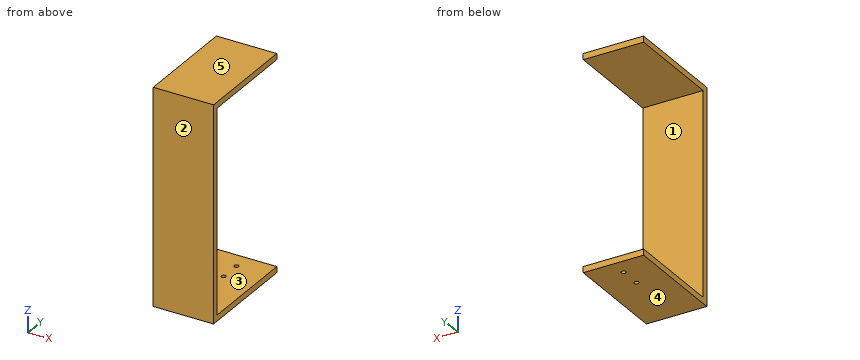
Autodesk Inventor part; units mm, degrees
ref_plane "YZ Plane" through (0, 0, 0) normal (1, 0, 0) x (0, 1, 0)
ref_plane "XZ Plane" through (0, 0, 0) normal (0, 1, 0) x (-1, 0, 0)
ref_plane "XY Plane" through (0, 0, 0) normal (0, 0, 1) x (1, 0, 0)
sketch "Sketch1" plane through (0, 0, 0) normal (0, 1, 0) x (-1, 0, 0)
  line L0 (0, 0) -> (-20, 0)
  line L1 (-20, 0) -> (-20, -67.262)
  line L2 (-20, -67.262) -> (0, -67.262)
  line L3 (0, -67.262) -> (0, 0)
  dimension "d0" = 20
  dimension "d1" = 67.262
extrude "Extrusion1" add sketch "Sketch1" along normal blind 2
sketch "Sketch2" plane through (0, 0, 0) normal (0, 0, 1) x (1, 0, 0)
  line L0 (0, 0) -> (20, 0)
  line L1 (20, 0) -> (20, 35)
  line L2 (20, 35) -> (0, 35)
  line L3 (0, 35) -> (0, 0)
  dimension "d4" = 20
  dimension "d5" = 35
extrude "Extrusion2" add sketch "Sketch2" along normal blind 2
sketch "Sketch4" plane through (20, 0, -67.262) normal (0, 0, -1) x (-1, 0, 0)
  line L0 (0, 35) -> (20, 35)
  line L1 (0, 35) -> (20, 35)
  line L2 (20, 35) -> (20, 0)
  line L3 (20, 0) -> (0, 0)
  line L4 (0, 0) -> (0, 35)
extrude "Extrusion3" add sketch "Sketch4" along normal blind 2
sketch "Sketch5" plane through (20, 0, -69.262) normal (0, 0, -1) x (-1, 0, 0)
  circle A0 centre (10, 29.36) radius 0.75
  line L0 (20, 35) -> (0, 35)
  line L1 (0, 35) -> (0, 0)
  point P0 (20, 0)
  dimension "d10" = 1.5
  dimension "d11" = 5.64
  dimension "d12" = 10
extrude "Extrusion4" cut sketch "Sketch5" against normal blind 2
sketch "Sketch6" plane through (20, 0, -69.262) normal (0, 0, -1) x (-1, 0, 0)
  circle A0 centre (10, 22.26) radius 0.75
  line L0 (0, 35) -> (0, 0)
  circle A1 centre (10, 29.36) radius 0.75
  point P0 (20, 0)
  dimension "d15" = 1.5
  dimension "d16" = 10
  dimension "d17" = 7.1
extrude "Extrusion5" cut sketch "Sketch6" against normal blind 2 contours A0
properties part number "Leg Servo Holder"
The model under review builds one solid part; all positions refer to its coordinate system, in mm. Face numbers are marked on the shaded views. A direction names the side the tool comes from. Round coordinates to 2 decimals unless told otherwise and drop trailing zeros. Loops run counter-clockwise (first coordinate to the right, second up) from the corner with the lowest first, then second, coordinate; pieces in that order, holes last. Notation, with made-up numbers: (80, -37) -> (101, -37) arc R17 cw to (101, -7) -> close; hole circle Ø7 at (81.5, 70). An arc over 180 degrees is marked (long way). Answer as a JSON object with one key per item and string values. Group by question number.
1) We need section C-C on x = 10. Write out the cut boundary in (y, z), then the cut area to 3 significant figures.
2) We need section B-B on y = 27. Write out the cut boundary in (x, z).
3) For line 1 (Y direction, x = 10, z = -68.6); line 2 (Z direction, x = 3, y = 10); line 3 (Y direction, x = 19.25, z = -60), list the stretches that pass through material, from the lowest coordinate up. Write a range as [from, to].
4) For the marked faces 1 and 2, list the 3-axis set-ups (+Z, -Z, +X, -X, +Y, -Y) from which the entire face can be reached by the end or side of a thin tool; tool diameter is ignored.
5) Mouldability with a two-part tool opening along Z and no side actions: class the marked faces 3, 4 and 5 as released by +Z, released by -Z, zero draft, split by the parting line, or undercut.
6) For pin 1 Ø5 at (x, z) = (17.5, -31.5) entering from +Y; pin 2 Ø1.7 at (x, y) = (10, 22.26) entering from -Z, all flat-tipped, find the tip position at first contact; note any pin that passes through.
7) We need section D-D on x = 17. Write out the cut boundary in (y, z).
8) We need section A-A on y = 22.26. Write out the cut boundary in (x, z), then the cut area to 3 significant figures.
Result set:
{
 "1": {"outline": "(0, -69.26) -> (21.51, -69.26) -> (21.51, -67.26) -> (2, -67.26) -> (2, 0) -> (35, 0) -> (35, 2) -> (0, 2) -> close; (23.01, -69.26) -> (28.61, -69.26) -> (28.61, -67.26) -> (23.01, -67.26) -> close; (30.11, -69.26) -> (35, -69.26) -> (35, -67.26) -> (30.11, -67.26) -> close", "area": "269 mm²"},
 "2": {"outline": "(0, -69.26) -> (20, -69.26) -> (20, -67.26) -> (0, -67.26) -> close; (0, 0) -> (20, 0) -> (20, 2) -> (0, 2) -> close"},
 "3": {"line 1": "[0, 21.51], [23.01, 28.61], [30.11, 35]", "line 2": "[-69.26, -67.26], [0, 2]", "line 3": "[0, 2]"},
 "4": {"face 1": "+X, -X, +Y", "face 2": "+Z, -Z, +X, -X, -Y"},
 "5": {"face 3": "undercut", "face 4": "released by -Z", "face 5": "released by +Z"},
 "6": {"pin 1": "y = 2", "pin 2": "z = -69.26"},
 "7": {"outline": "(0, -69.26) -> (35, -69.26) -> (35, -67.26) -> (2, -67.26) -> (2, 0) -> (35, 0) -> (35, 2) -> (0, 2) -> close"},
 "8": {"outline": "(0, -69.26) -> (9.25, -69.26) -> (9.25, -67.26) -> (0, -67.26) -> close; (0, 0) -> (20, 0) -> (20, 2) -> (0, 2) -> close; (10.75, -69.26) -> (20, -69.26) -> (20, -67.26) -> (10.75, -67.26) -> close", "area": "77.0 mm²"}
}
